Part model, mm, in its own coordinate system. Round coordinates to 2 decimals unless told otherwise and drop trailing zeros. Answer as a JSON object with one key per item and string values. Group by question number.
from build123d import *

# Parameters (mm, degrees)
SKETCH_1_R          = 125
EXTRUDE_1_DEPTH     = 6
SKETCH_3_R          = 3
CUT_EXTRUDE_2_DEPTH = 10
SKETCH_4_R          = 2.5
CUT_EXTRUDE_3_DEPTH = 10
CHAMFER_1_SIZE      = 1


with BuildPart() as part:
    # Эскиз1 → Бобышка-Вытянуть1 (new body)
    with BuildSketch(Plane(origin=(0, 0, 0), x_dir=(1, 0, 0), z_dir=(0, 1, 0))):
        with Locations(Location((0, 0, 0), (0, 0, 270))):
            Circle(SKETCH_1_R)
    extrude(amount=EXTRUDE_1_DEPTH)

    # Эскиз3 → Вырез-Вытянуть2 (cut)
    with BuildSketch(Plane(origin=(0, 6, 0), x_dir=(1, 0, 0), z_dir=(0, 1, 0))):
        with Locations(Location((0, 112.5, 0), (0, 0, 270))):
            Circle(SKETCH_3_R)
        with Locations(Location((-112.5, 0, 0), (0, 0, 270))):
            Circle(SKETCH_3_R)
        with Locations(Location((0, -112.5, 0), (0, 0, 270))):
            Circle(SKETCH_3_R)
        with Locations(Location((112.5, 0, 0), (0, 0, 270))):
            Circle(SKETCH_3_R)
    extrude(amount=-CUT_EXTRUDE_2_DEPTH, mode=Mode.SUBTRACT)

    # Эскиз4 → Вырез-Вытянуть3 (cut)
    with BuildSketch(Plane.XZ):
        with Locations(Location((0, 62.5, 0), (0, 0, 270))):
            Circle(SKETCH_4_R)
        with Locations(Location((0, -62.5, 0), (0, 0, 270))):
            Circle(SKETCH_4_R)
        with Locations(Location((62.5, 0, 0), (0, 0, 270))):
            Circle(SKETCH_4_R)
        with Locations(Location((-62.5, 0, 0), (0, 0, 270))):
            Circle(SKETCH_4_R)
    extrude(amount=-CUT_EXTRUDE_3_DEPTH, mode=Mode.SUBTRACT)

    # Фаска1
    chamfer_1_edges = [part.edges().sort_by_distance(p)[0] for p in [
        (0, 6, -125),
    ]]
    chamfer(chamfer_1_edges, length=CHAMFER_1_SIZE)


solid = part.part
Item 1: Drill centre lines: line 1 (X direction, y = 1.4, z = 0); line 2 (Z direction, x = -69, y = 2.05); line 3 (X direction, y = 3.6, z = 29.5). Where is each one in solid material? Low to high.
Item 2: Band-saw the part on A-A, the plane y = 3.25. Count the separate pieces of the cut face and the enclosed holes in it, plus the area to 3 significant figures.
Item 3: Two-plate mould, pull along X, no slides. Class faces 1 (the face through (0.9, 3.04, 115.36)), 2 (the face through (2, 6, -2)), 3 (the face through (5.5, 2.46, -124.88)): pulls with the +X half, pulls with the -X half, needs draft (parallel to the pull), parting line crosses it, or undercut.
Item 4: Drop flat-ended pins along their axis: pin 1 Ø9.5 at (x, z) = (0, -112.5) entering from +Y; pin 2 Ø4.5 at (x, z) = (0, -62.5) entering from +Y; pin 3 Ø3 at (x, y) = (92.5, 5) entering from +Z. Give the stop position or say it passes through.
Entries:
{
 "1": {"line 1": "-125 to -115.5, -109.5 to -65, -60 to 60, 65 to 109.5, 115.5 to 125", "line 2": "-104.23 to 104.23", "line 3": "-121.47 to 121.47"},
 "2": {"separate pieces": "1", "enclosed holes": "8", "area": "48,900 mm²"},
 "3": {"face 1": "undercut", "face 2": "needs draft", "face 3": "parting line crosses it"},
 "4": {"pin 1": "y = 6", "pin 2": "through", "pin 3": "z = 85.7"}
}
